The listing builds one solid part. Answer for the finished solid, in the listing's coordinates (mm). A direction names the side the tool comes from. Coordinates: 2 decimals unless noted, no trailing zeros. Order: outer loops, then holes, each group sorted by start corner. A loop starts at its lowest first (then second) coordinate and runs counter-clockwise, first axis right, second up.
Autodesk Inventor part; units mm, degrees
ref_plane "YZ Plane" through (0, 0, 0) normal (1, 0, 0) x (0, 1, 0)
ref_plane "XZ Plane" through (0, 0, 0) normal (0, 1, 0) x (-1, 0, 0)
ref_plane "XY Plane" through (0, 0, 0) normal (0, 0, 1) x (1, 0, 0)
sketch "Sketch1" plane through (0, 0, 0) normal (0, 0, 1) x (1, 0, 0)
  line L0 (-48, 48) -> (48, 48) construction
  line L1 (48, 48) -> (48, -48) construction
  line L2 (48, -48) -> (-48, -48) construction
  line L3 (-48, -48) -> (-48, 48) construction
  circle A0 centre (-45, 45) radius 2.25
  circle A1 centre (45, 45) radius 2.25
  line L4 (45, 45) -> (-45, 45) construction
  line L5 (-45, 45) -> (-45, -45) construction
  line L6 (-45, -45) -> (45, -45) construction
  line L7 (45, -45) -> (45, 45) construction
  circle A2 centre (45, -45) radius 2.25
  circle A3 centre (-45, -45) radius 2.25
  line L8 (-50.5, -50.5) -> (-42, -50.5)
  line L9 (-42, -50.5) -> (-42, -42)
  line L10 (-42, -42) -> (-50.5, -42)
  line L11 (-50.5, -42) -> (-50.5, -50.5)
  line L12 (0, 0) -> (-48, -48) construction
  line L13 (-30, 36.5) -> (30, 36.5)
  line L14 (30, 36.5) -> (30, -36.5)
  line L15 (30, -36.5) -> (-30, -36.5)
  line L16 (-30, -36.5) -> (-30, 36.5)
  line L17 (-2.4749, 2.4749) -> (2.4749, -2.4749)
  line L18 (2.4749, -2.4749) -> (-42.5251, -47.4749)
  line L19 (-42.5251, -47.4749) -> (-47.4749, -42.5251)
  line L20 (-47.4749, -42.5251) -> (-2.4749, 2.4749)
  line L21 (0, 0) -> (-45, -45) construction
  point P0 (0, 48)
  point P1 (48, 0)
  point P2 (30, 0)
  point P3 (0, 36.5)
  dimension "d0" = 96
  dimension "d1" = 96
  dimension "d2" = 4.5
  dimension "d3" = 4.5
  dimension "d4" = 3
  dimension "d5" = 4.5
  dimension "d6" = 4.5
  dimension "d9" = 3
  dimension "d10" = 3
  dimension "d11" = 60
  dimension "d12" = 73
  dimension "d13" = 7
  dimension "d14" = 0
  dimension "d23" = 5.5
  dimension "d24" = 5.5
extrude "Extrusion1" add sketch "Sketch1" along normal blind 1.5 contours L20 L17 L18 L16 | L16 L13 L14 L15 L18 L17 L20
extrude "Extrusion2" add sketch "Sketch1" along normal blind 1.5 contours A3 L19 | A3 L19 L20 L10 L9 L18 | A3 L19 L18 L9 L8 L11 L10 L20 | L20 L16 L18 L9 L10 | L20 L17 L18 L16 picked at (-45.2318, -44.2867)
extrude "Extrusion3" cut sketch "Sketch1" along normal blind 10 contours A3 L19 | L19 A3
mirror "Mirror1" about plane through (0, 0, 0) normal (1, 0, 0) of "Extrusion2", "Extrusion3"
mirror "Mirror2" about plane through (0, 0, 0) normal (0, 1, 0) of "Extrusion2", "Extrusion3", "Mirror1"
fillet "Fillet1" radius 2 4 edges at (-30, 34.9497, 0.75) (30, 34.9497, 0.75) (30, -34.9497, 0.75) (-30, -34.9497, 0.75)
fillet "Fillet2" radius 5 4 edges at (-30, -25.0503, 0.75) (-30, 25.0503, 0.75) (30, 25.0503, 0.75) (30, -25.0503, 0.75)
properties part number "BattHolder"
(1) Find section C-C on x = 33.5. Determine the outline of the cut face in (y, z), then the cut area to 3 significant figures.
(2) The mould has two halves that part along X. Classify faces 5 (the flat face through (39.32, 34.37, 0.74)), 6 (the flat face through (-39.1, 34.15, 0.74)), 7 (the cylindrical face through (-46.66, 43.48, 0.74)): pulls with the +X half, pulls with the -X half, needs draft (parallel to the pull), parting line crosses it, or undercut.
(3) Find section A-A on x = -45. Determine the outline of the cut face in (y, z).
(4) Find the intervals of material crossed by probe 1 along X at (y, z) = (-45, 0.6); probe 2 along Y at (x, z) = (22, 0.85), in increasing order.
(5) A tool of negligible diameter and unlimited length cuts with its end or side. For faces 1 (the flat face through (-39.32, -34.37, 0.74)), 2 (the flat face through (39.1, -34.15, 0.74)), 3 (the flat face through (36.95, 41.9, 0.74)), 4 (the flat face through (-36.95, -41.9, 0.74)), from which of +Z, -Z, +X, -X, +Y, -Y can it reach the whole face along a straight path? Write none if from no direction.
(6) Find section D-D on z = 1. Count the separate pieces of the cut face and the enclosed holes in it, then the cut area to 3 significant figures.
(7) Find section B-B on y = 38.5. Determine the outline of the cut face in (x, z), then the cut area to 3 significant figures.
Resolved:
1. outline: (-38.45, 0) - (-28.55, 0) - (-28.55, 1.5) - (-38.45, 1.5) - close; (28.55, 0) - (38.45, 0) - (38.45, 1.5) - (28.55, 1.5) - close
1. area: 29.7 mm2
2. face 5: pulls with the +X half
2. face 6: pulls with the -X half
2. face 7: undercut
3. outline: (-50.5, 0) - (-47.25, 0) - (-47.25, 1.5) - (-50.5, 1.5) - close; (-42.75, 0) - (-40.05, 0) - (-40.05, 1.5) - (-42.75, 1.5) - close; (40.05, 0) - (42.75, 0) - (42.75, 1.5) - (40.05, 1.5) - close; (47.25, 0) - (50.5, 0) - (50.5, 1.5) - (47.25, 1.5) - close
4. probe 1: x = -50.5 to -47.25, -42.75 to -40.05, 40.05 to 42.75, 47.25 to 50.5
4. probe 2: y = -36.5 to 36.5
5. face 1: +Z, -Z, -X
5. face 2: +Z, -Z, +X
5. face 3: +Z, -Z, +Y
5. face 4: +Z, -Z, -Y
6. separate pieces: 1
6. enclosed holes: 4
6. area: 5,140 mm2
7. outline: (-43.45, 0) - (-33.55, 0) - (-33.55, 1.5) - (-43.45, 1.5) - close; (33.55, 0) - (43.45, 0) - (43.45, 1.5) - (33.55, 1.5) - close
7. area: 29.7 mm2
